from build123d import *

# Parameters (mm, degrees)
F0_W     = 70
F0_H     = 70
F0_R     = 20
F1_DEPTH = 2
F2_DEPTH = 1


# Not quite as in the source:
# - a feature names something its author has since deleted; it is built from what else it names


with BuildPart() as f1:
    # F0 (on Top) → F1 (new body)
    with BuildSketch(Plane.XY):
        Rectangle(F0_W, F0_H)
        Circle(F0_R, mode=Mode.SUBTRACT)
    extrude(amount=F1_DEPTH)



with BuildPart() as f1b:
    # F0 (on Top) → F1, piece 2 (new body)
    with BuildSketch(Plane.XY):
        Polygon((10.3923048454, 6), (-10.3923048454, 6), (0, -12), align=None)
    extrude(amount=F1_DEPTH)


with BuildPart() as f1_1:
    add(f1.part)

    add(f1b.part)  # F2 merges F1b
    # F0 (on Top) → F2 (join)
    with BuildSketch(Plane.XY):
        Rectangle(F0_W, F0_H)
        Circle(F0_R, mode=Mode.SUBTRACT)
        Circle(F0_R)
        Polygon((0, -12), (-10.3923048454, 6), (10.3923048454, 6), align=None, mode=Mode.SUBTRACT)
        Polygon((10.3923048454, 6), (-10.3923048454, 6), (0, -12), align=None)
    extrude(amount=-F2_DEPTH)


solid = f1_1.part
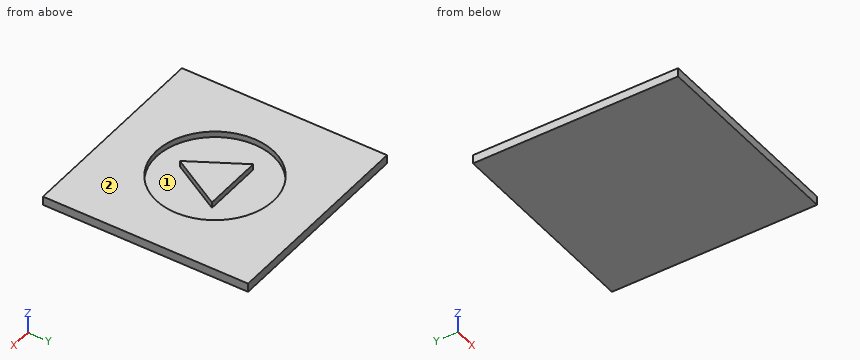
The listing builds one solid part. Answer for the finished solid, in the listing's coordinates (mm). Face numbers are marked on the shaded views. Give positions to 0.01 mm unless a question says otherwise; leave off trailing zeros. Loops run counter-clockwise (first coordinate to the right, second up) from the corner with the lowest first, then second, coordinate; pieces in that order, holes last.
Item 1: A cutting plane is placed at D-D (x = 7). Give the vertices of the cut face in (y, z) (3 decimals).
Derived:
outline: (-35, -1) - (35, -1) - (35, 2) - (18.735, 2) - (18.735, 0) - (6, 0) - (6, 2) - (0.124, 2) - (0.124, 0) - (-18.735, 0) - (-18.735, 2) - (-35, 2) - close
Item 2: Determine the mould class of the marked faces 1 and 2 for opening direction X: +X half, -X half, draft (parallel to the pull), parting line (faces both ways), or undercut.
Derived:
face 1: undercut
face 2: draft
Item 3: A cutting plane is placed at B-B (x = 16). Give the vertices of the cut face in (y, z), then the cut area to 3 significant figures.
Derived:
outline: (-35, -1) - (35, -1) - (35, 2) - (12, 2) - (12, 0) - (-12, 0) - (-12, 2) - (-35, 2) - close
area: 162 mm2
Item 4: A cutting plane is placed at C-C (y = -17). Give the vertices of the cut face in (x, z), then the cut area to 3 significant figures.
Derived:
outline: (-35, -1) - (35, -1) - (35, 2) - (10.54, 2) - (10.54, 0) - (-10.54, 0) - (-10.54, 2) - (-35, 2) - close
area: 168 mm2
Item 5: A cutting plane is placed at A-A (z = 0.45). Give the vertices of the cut face in (x, y), then the cut area to 3 significant figures.
Derived:
outline: (-35, -35) - (35, -35) - (35, 35) - (-35, 35) - close; (-10.39, 6) - (0, -12) - (10.39, 6) - close; hole circle Ø40 at (0, 0)
area: 3,830 mm2
Item 6: Find the intervals of material crossed by line 1 along X through (y, z) = (-4, 0.3); line 2 along X through (y, z) = (-9.5, 0.6); line 3 along Z through (x, y) = (1.5, -19), in increasing order.
Derived:
line 1: x = -35 to -19.6, -4.62 to 4.62, 19.6 to 35
line 2: x = -35 to -17.6, -1.44 to 1.44, 17.6 to 35
line 3: z = -1 to 0
